Verification items for the finished model (mm, model axes). A direction names the side the tool comes from. Give positions to 0.01 mm unless a question says otherwise; leave off trailing zeros. Write each loop counter-clockwise with the first axis right and the second up, starting at its lowest first coordinate (ties: lowest second). Pieces come first, ordered by that corner, then holes. Notation, with made-up numbers: (74.25, 2) -> (102.25, 2) arc R17 ccw to (102.25, 34) -> close; hole circle Ø11 at (34.5, 59.25). An arc over 180 degrees is marked (long way). Answer as CSV lines item,"result". Start each with the question number.
1) Sectioned sample at D-D on y = 9.5. Record the cut outline in (x, z).
2) Sectioned sample at A-A on x = 0. Record the cut outline in (y, z).
3) Sectioned sample at C-C on z = 4.5. Record the cut outline in (x, y), and give its area (3 significant figures).
4) Mould release check, pull along Z, two halves, no side actions. Record for faces 4 (the flat face through (14, 14, 27)), 5 (the cylindrical face through (14.199, 42.862, 11.753)), 6 (the cylindrical face through (14.2, -15.29, 21.47)), 7 (the cylindrical face through (10.35, 14.26, 3.45)): released by +Z, released by -Z, zero draft, split by the parting line, or undercut.
5) Tool access check on faces 1 (the cylindrical face through (-10.35, 14.32, 3.45)), 2 (the flat face through (-2, 23, 7)), 3 (the flat face through (-15.75, 13, 3)). Record the directions out of +Z, -Z, +X, -X, +Y, -Y that give a thin tool (end or side, any length) a straight path to the whole face; none if there is none.
6) Sectioned sample at B-B on x = 5.5. Record the cut outline in (y, z).
7) Material ranges on L1, parallel to Y at x = 0, z = 5.25; L2, parallel to Z at x = 14, y = 16.5; L3, parallel to X at y = 42.5, z = 10.5, recorded low to high.
8) Gauge pin test, flat ends, axial feed: pin 1 Ø4 at (y, z) = (16.7, 22.9) entering from +X; pin 2 Ø8.5 at (x, y) = (1, 24.5) entering from +Z; pin 3 Ø10 at (y, z) = (0, 17) entering from -X. Record the tip position at first contact, or that the pin passes through.
```python
from build123d import *

# Parameters (mm, degrees)
SKETCH_1_W      = 31.500863908
SKETCH_1_H      = 80
SKETCH_1_R      = 10.417524335
SKETCH_1_R_2    = 1.56
EXTRUDE_1_DEPTH = 7
SKETCH_5_W      = 3.14774975
SKETCH_5_H      = 80
EXTRUDE_2_DEPTH = 27
MM_1_D          = 3
MM_1_DEPTH      = 3.14774975


with BuildPart() as part:
    # 草图1 → 凸台-拉伸1 (new body)
    with BuildSketch(Plane.XY):
        with Locations((0, 13.377078694)):
            Rectangle(SKETCH_1_W, SKETCH_1_H)
        with Locations((0, -6.708333333)):
            Circle(SKETCH_1_R, mode=Mode.SUBTRACT)
        with Locations((0, -20.208333333)):
            Circle(SKETCH_1_R_2, mode=Mode.SUBTRACT)
        with BuildLine():
            Line((8.85, 15.791666667), (-8.85, 15.791666667))
            ThreePointArc((-8.85, 15.791666667), (-10.35, 14.291666667), (-8.85, 12.791666667))
            Line((-8.85, 12.791666667), (8.85, 12.791666667))
            ThreePointArc((8.85, 12.791666667), (10.35, 14.291666667), (8.85, 15.791666667))
        make_face(mode=Mode.SUBTRACT)
    extrude(amount=EXTRUDE_1_DEPTH)

    # 草图5 → 凸台-拉伸2 (add)
    with BuildSketch(Plane.XY):
        with Locations((14.176557079, 13.377078694)):
            Rectangle(SKETCH_5_W, SKETCH_5_H)
    extrude(amount=EXTRUDE_2_DEPTH)

    # 大小mm 暗销孔1
    with Locations(Plane.ZY.offset(-12.602682204)):
        with Locations((12.444794173, 44.192540423), (23.673777791, 43.57849825), (11.130072788, -15.739218974), (22.900107862, -15.739218974), (12.444794173, 16.704513785), (22.900107862, 16.704513785)):
            Hole(MM_1_D / 2, depth=MM_1_DEPTH)


solid = part.part
```
Ans:
1,outline,"(-15.75, 0) -> (15.75, 0) -> (15.75, 27) -> (12.6, 27) -> (12.6, 7) -> (-15.75, 7) -> close"
2,outline,"(-26.62, 0) -> (-21.77, 0) -> (-21.77, 7) -> (-26.62, 7) -> close; (-18.65, 0) -> (-17.13, 0) -> (-17.13, 7) -> (-18.65, 7) -> close; (3.71, 0) -> (12.79, 0) -> (12.79, 7) -> (3.71, 7) -> close; (15.79, 0) -> (53.38, 0) -> (53.38, 7) -> (15.79, 7) -> close"
3,outline,"(-15.75, -26.62) -> (15.75, -26.62) -> (15.75, 53.38) -> (-15.75, 53.38) -> close; hole circle Ø20.84 at (0, -6.71); hole (-8.85, 12.79) -> (8.85, 12.79) arc R1.5 ccw to (8.85, 15.79) -> (-8.85, 15.79) arc R1.5 ccw to start; hole circle Ø3.12 at (0, -20.21)"
3,area,"2,110 mm²"
4,face 4,"released by +Z"
4,face 5,"undercut"
4,face 6,"undercut"
4,face 7,"zero draft"
5,face 1,"+Z, -Z"
5,face 2,"+Z, -X, +Y, -Y"
5,face 3,"+Z, -Z, -X, +Y, -Y"
6,outline,"(-26.62, 0) -> (-15.56, 0) -> (-15.56, 7) -> (-26.62, 7) -> close; (2.14, 0) -> (12.79, 0) -> (12.79, 7) -> (2.14, 7) -> close; (15.79, 0) -> (53.38, 0) -> (53.38, 7) -> (15.79, 7) -> close"
7,L1,"y = -26.62 to -21.77, -18.65 to -17.13, 3.71 to 12.79, 15.79 to 53.38"
7,L2,"z = 0 to 10.96, 13.93 to 21.41, 24.39 to 27"
7,L3,"x = 12.6 to 15.75"
8,pin 1,"stops at x = 15.75"
8,pin 2,"stops at z = 7"
8,pin 3,"stops at x = 12.6"
